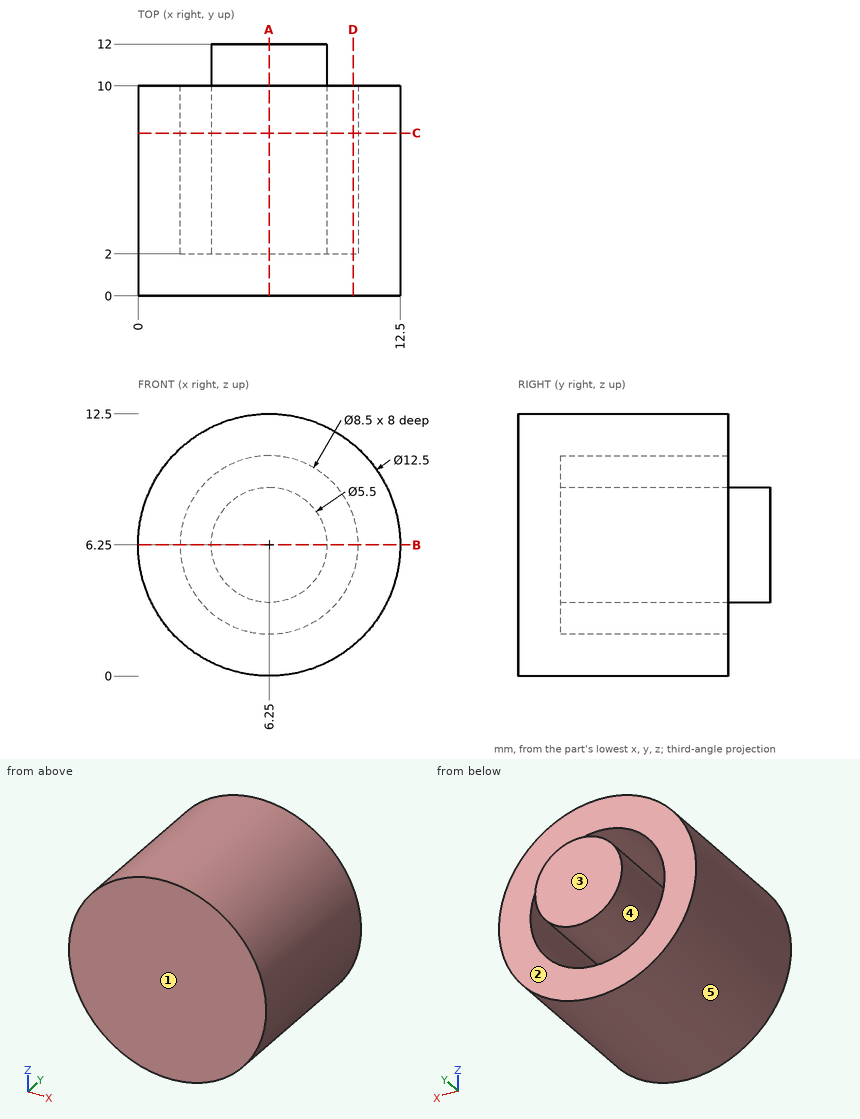
Verification items for this drawing (mm, ordinates from the low corner). A direction names the side the tool comes from. Round coordinates to 2 decimals unless told otherwise and drop trailing zeros. Loops run counter-clockwise (first coordinate to the right, second up) from the corner with the lowest first, then second, coordinate; pieces in that order, holes last. Notation, with made-up numbers: (72.5, 54) - (120.5, 54) arc R21 cw to (120.5, 68) - close; hole circle Ø7 at (69.25, 12.25). An arc over 180 degrees is marked (long way). Write item = value, one per line.
Q1. Sectioned sample at B-B on z = 6.25. Record the boundary of the cut face in (x, y).
Here are the results:
outline = (0, 0) - (12.5, 0) - (12.5, 10) - (10.5, 10) - (10.5, 2) - (9, 2) - (9, 12) - (3.5, 12) - (3.5, 2) - (2, 2) - (2, 10) - (0, 10) - close
Q2. Mould release check, pull along Z, two halves, no side actions. Record for the marked faces 3, 4 and 5: +Z half, -Z half, draft (parallel to the pull), parting line (faces both ways), or undercut.
Here are the results:
face_3 = draft
face_4 = undercut
face_5 = parting line
Q3. Material ranges on L1, parallel to X at y = 8.25, z = 6.25; L2, parallel to Z at x = 4, y = 6.25; L3, parallel to Y at x = 3, z = 11.25, recorded low to high.
Here are the results:
L1 = 0 to 2, 3.5 to 9, 10.5 to 12.5
L2 = 0.42 to 2.64, 4.67 to 7.83, 9.86 to 12.08
L3 = 0 to 10
Q4. Sectioned sample at D-D on x = 10.25. Record the boundary of the cut face in (y, z), plus the area to 3 significant figures.
Here are the results:
outline = (0, 1.45) - (10, 1.45) - (10, 4.81) - (2, 4.81) - (2, 7.69) - (10, 7.69) - (10, 11.05) - (0, 11.05) - close
area = 73.1 mm^2
Q5. Sectioned sample at A-A on x = 6.25. Record the boundary of the cut face in (y, z).
Here are the results:
outline = (0, 0) - (10, 0) - (10, 2) - (2, 2) - (2, 3.5) - (12, 3.5) - (12, 9) - (2, 9) - (2, 10.5) - (10, 10.5) - (10, 12.5) - (0, 12.5) - close
Q6. Sectioned sample at C-C on y = 7.75. Record the boundary of the cut face in (x, z), plus the area to 3 significant figures.
Here are the results:
outline = circle Ø12.5 at (6.25, 6.25); circle Ø5.5 at (6.25, 6.25); hole circle Ø8.5 at (6.25, 6.25)
area = 89.7 mm^2
Q7. Tool access check on the marked faces 1 and 2. Record the directions out of +Z, -Z, +X, -X, +Y, -Y that give a thin tool (end or side, any length) a straight path to the whole face; none if there is none.
Here are the results:
face_1 = +Z, -Z, +X, -X, -Y
face_2 = +Y
Q8. Depth check by flat-ended pin: pin 1 (2 mm diameter, centred on x = 10, z = 9.5, fed in from +Y); pin 2 (4 mm diameter, centred on y = 7.5, z = 10, fed in from -X). Enter the tip coordinate at first touch or a pass-through.
Here are the results:
pin_1 = 10
pin_2 = 0.25
